Build history of the part. All positions in model axes, mm. Face numbers are marked on the shaded views. A direction names the side the tool comes from. Give positions to 0.01 mm unless a question says otherwise; leave off trailing zeros. Order: outer loops, then holes, each group sorted by start corner. A loop starts at its lowest first (then second) coordinate and runs counter-clockwise, first axis right, second up. Notation, with made-up numbers: (52, 67) -> (85, 67) arc R33 ccw to (85, 97) -> close; hole circle Ø5 at (78, 73.5). An arc over 180 degrees is marked (long way). One line per question, with ' | ' between items. Start each with the question number.
(1) Cut at A-A (x = 3). Give the cut face in (y, z), then the cut area to 3 significant figures.
(2) Drill centre lines: L1, parallel to X at y = 35.5, z = 14; L2, parallel to Y at x = 6.5, z = 15.5; L3, parallel to Y at x = 7, z = 21. Where is each one in solid material? Low to high. Write a range as from..to.
(3) Cut at C-C (z = 18.25). Give the cut face in (x, y).
(4) Cut at B-B (y = 30.5). Give the cut face in (x, z).
(5) Which spindle directions (+Z, -Z, +X, -X, +Y, -Y) get a long thin tool onto all of the face, cutting with end or side? Do the marked faces 1, 2, 3 and 4. Say none if no direction does.
(6) Pin check, flat tips, straight feed: pin 1 Ø5 at (y, z) = (8.5, 10.5) entering from -X; pin 2 Ø7.5 at (y, z) = (38.5, 15.5) entering from -X; pin 3 Ø8 at (y, z) = (43, 21.5) entering from +X; pin 4 Ø9.5 at (x, z) = (37.5, 12) entering from +Y. Stop position of each tip, or through.
(7) Cut at D-D (x = 20). Give the cut face in (y, z), then the cut area to 3 significant figures.
from build123d import *

# Parameters (mm, degrees)
F1_DEPTH = 25.4
F2_SIZE  = 5.08
F3_SIZE  = 5.08
F4_R     = 5.08
F5_SIZE  = 5.08
F6_SIZE  = 5.08


with BuildPart() as f1:
    # F0 (on Top) → F1 (new body)
    with BuildSketch(Plane.XY):
        Polygon((0, 31.75), (0, 0), (44.45, 0), (44.45, 31.75), (32.315474, 31.75), (32.315474, 60.153503), (21.024525, 60.153503), (9.733576, 60.153503), (9.733576, 31.75), align=None)
    extrude(amount=F1_DEPTH)

    # F2
    f2_edges = [f1.edges().sort_by_distance(p)[0] for p in [
        (4.866788, 31.75, 25.4),
    ]]
    chamfer(f2_edges, length=F2_SIZE)

    # F3
    f3_edges = [f1.edges().sort_by_distance(p)[0] for p in [
        (4.866788, 31.75, 0),
    ]]
    chamfer(f3_edges, length=F3_SIZE)

    # F4
    f4_edges = [f1.edges().sort_by_distance(p)[0] for p in [
        (38.382737, 31.75, 25.4),
    ]]
    fillet(f4_edges, radius=F4_R)

    # F5
    f5_edges = [f1.edges().sort_by_distance(p)[0] for p in [
        (38.382737, 31.75, 0),
    ]]
    chamfer(f5_edges, length=F5_SIZE)

    # F6
    f6_edges = [f1.edges().sort_by_distance(p)[0] for p in [
        (32.315474, 60.153503, 12.7),
        (21.024525, 60.153503, 25.4),
        (9.733576, 60.153503, 12.7),
        (21.024525, 60.153503, 0),
    ]]
    chamfer(f6_edges, length=F6_SIZE)


solid = f1.part
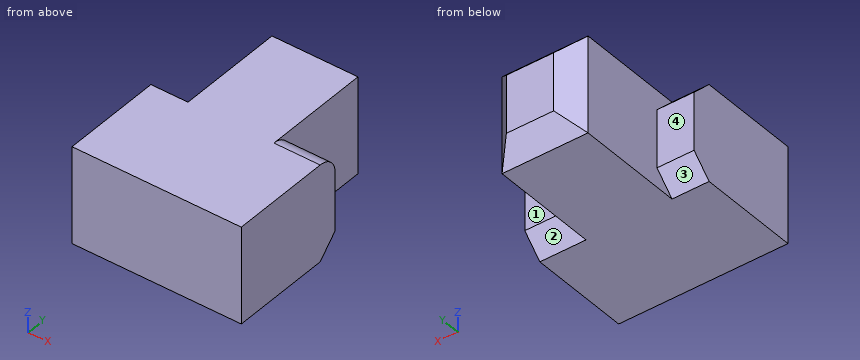
Result set:
1) outline: (0, 0) -> (26.67, 0) -> (31.75, 5.08) -> (31.75, 20.32) -> (26.67, 25.4) -> (0, 25.4) -> close | area: 781 mm2
2) L1: x = 9.73..32.32 | L2: y = 0..31.75 | L3: y = 0..31.07
3) outline: (0, 0) -> (44.45, 0) -> (44.45, 31.75) -> (32.32, 31.75) -> (32.32, 55.07) -> (27.24, 60.15) -> (14.81, 60.15) -> (9.73, 55.07) -> (9.73, 31.75) -> (0, 31.75) -> close
4) outline: (0, 3.83) -> (9.73, 3.83) -> (9.73, 0) -> (32.32, 0) -> (32.32, 3.83) -> (44.45, 3.83) -> (44.45, 23.66) -> (32.32, 23.66) -> (32.32, 25.4) -> (9.73, 25.4) -> (9.73, 21.57) -> (0, 21.57) -> close
5) face 1: +Z, -Z, +X, +Y | face 2: -Z, +X, +Y | face 3: -Z, -X, +Y | face 4: +Z, -Z, -X, +Y
6) pin 1: stops at x = 0 | pin 2: stops at x = 9.73 | pin 3: stops at x = 32.32 | pin 4: stops at y = 31.75
7) outline: (0, 0) -> (55.07, 0) -> (60.15, 5.08) -> (60.15, 20.32) -> (55.07, 25.4) -> (0, 25.4) -> close | area: 1,500 mm2
